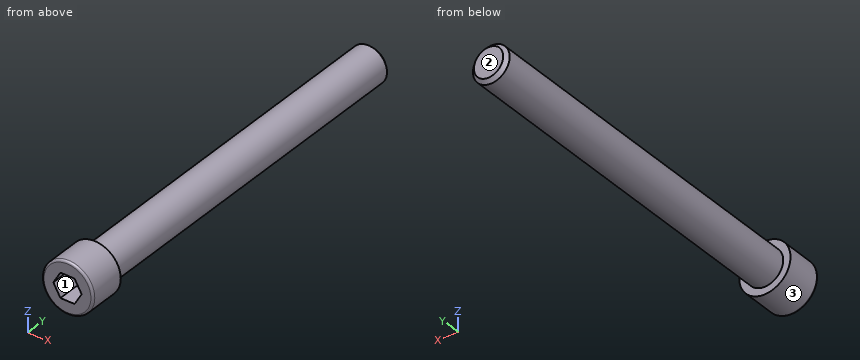
Solid Edge part; units mm, degrees
sketch "Sketch1" plane through (0, 0, 0) normal (0, -1, 0) x (1, 0, 0)
  circle A0 centre (0, 0) radius 2.5
extrude "Protrusion1" add sketch "Sketch1" against normal blind 50
sketch "Sketch2" plane through (0, 0, 0) normal (0, -1, 0) x (1, 0, 0)
  circle A0 centre (0, 0) radius 3.5
extrude "ExtrudedProtrusion_2" add sketch "Sketch2" along normal blind 5
fillet "Round_1" radius 0.3 1 edges at (-3.5, -5, 0)
chamfer "Chamfer_1" distance 0.5 angle 45 1 edges at (-2.5, 50, 0) measured on face at (-1.6167, 50, 1.7167)
sketch "Sketch3" plane through (0, -5, 0) normal (0, -1, 0) x (1, 0, 0)
  line L0 (-0.9646, 1.6708) -> (-1.9293, 0)
  line L1 (-1.9293, 0) -> (-0.9646, -1.6708)
  line L2 (-0.9646, -1.6708) -> (0.9646, -1.6708)
  line L3 (0.9646, -1.6708) -> (1.9293, 0)
  line L4 (1.9293, 0) -> (0.9646, 1.6708)
  line L5 (0.9646, 1.6708) -> (-0.9646, 1.6708)
extrude "ExtrudedCutout_1" cut sketch "Sketch3" along normal mid plane 8
cosmetic_thread "Thread1"
Work out the finished part from the listing and answer in its coordinate system (mm). Face numbers are marked on the shaded views. Give positions to 0.01 mm unless a question says otherwise; leave off trailing zeros. Write each loop counter-clockwise with the first axis right and the second up, starting at its lowest first coordinate (ties: lowest second). Pieces come first, ordered by that corner, then holes. Notation, with made-up numbers: (68, -27) - (118, -27) arc R24 cw to (118, -2) - close; hole circle Ø2 at (62.5, 70.5). An arc over 180 degrees is marked (long way). One line per item, written item: value. Start each with the question number.
1. For a pull along Z with two mould halves and no side action, classify the marked faces 1, 2 and 3 as +Z half, -Z half, draft (parallel to the pull), parting line (faces both ways), or undercut.
2. Find section A-A (x = 0). Write down the section's boundary in (y, z), then the cut area to 3 significant figures.
3. Find section B-B (y = 10.5). Write down the section's boundary in (x, z).
4. Given pin 1 (1 mm diameter, centred on x = 1.5, y = 20.5, fed in from -Z); pin 2 (4 mm diameter, centred on y = 9, z = 0, fed in from -X); pin 3 (1.5 mm diameter, centred on x = 2.5, z = 2.5, fed in from +Y), each flat-ended and moving along its own axis, determine where each tip first touches the part or whether it passes through.
5. Consider probe 1 along Y at (x, z) = (0, 1.25); probe 2 along Z at (x, y) = (0, 6); probe 3 along Y at (x, z) = (2.5, 1.5). Determine where each line is inside the solid, lowest interval first.
Geometry results:
1. face 1: undercut
1. face 2: draft
1. face 3: parting line
2. outline: (-5, -3.2) arc R0.3 ccw to (-4.7, -3.5) - (0, -3.5) - (0, -2.5) - (49.5, -2.5) - (50, -2) - (50, 2) - (49.5, 2.5) - (0, 2.5) - (0, 3.5) - (-4.7, 3.5) arc R0.3 ccw to (-5, 3.2) - (-5, 1.67) - (-1, 1.67) - (-1, -1.67) - (-5, -1.67) - close
2. area: 271 mm2
3. outline: circle Ø5 at (0, 0)
4. pin 1: z = -2.29
4. pin 2: x = -2.5
4. pin 3: y = 0
5. probe 1: -1 to 50
5. probe 2: -2.5 to 2.5
5. probe 3: -5 to 0
